Part print with two shaded views. Sizes in mm from the minimum x, y, z corner. Round coordinates to 2 decimals unless told otherwise and drop trailing zeros. Loops run counter-clockwise (first coordinate to the right, second up) from the corner with the lowest first, then second, coordinate; pieces in that order, holes last.
(1) Cut at A-A on y = 10. List the corners of the cut face in (x, z).
(2) Cut at D-D on y = 29. List the corners of the cut face in (x, z), then the cut area to 3 significant figures.
(3) Flat gauge pin, fed straight in: pin 1 (1 mm diameter, centred on y = 34, z = 2, fed in from +X). Where does the tip first touch, or does it go through?
(4) Mould opens along Y. For the marked faces 1, 2, 3 and 4 say: +Y half, -Y half, draft (parallel to the pull), parting line (faces both ways), or undercut.
(5) Cut at B-B on z = 2.85. Count the separate pieces of the cut face and the enclosed holes in it, then the cut area to 3 significant figures.
(6) Probe probe 1 along X at (y, z) = (12, 1.6); probe 2 along Y at (x, z) = (10, 2.85); probe 3 along Y at (x, z) = (16, 3.45). List the from-to ranges inside material, lowest first.
(7) Cut at C-C on x = 9.5. List the corners of the cut face in (y, z), then the cut area to 3 significant figures.
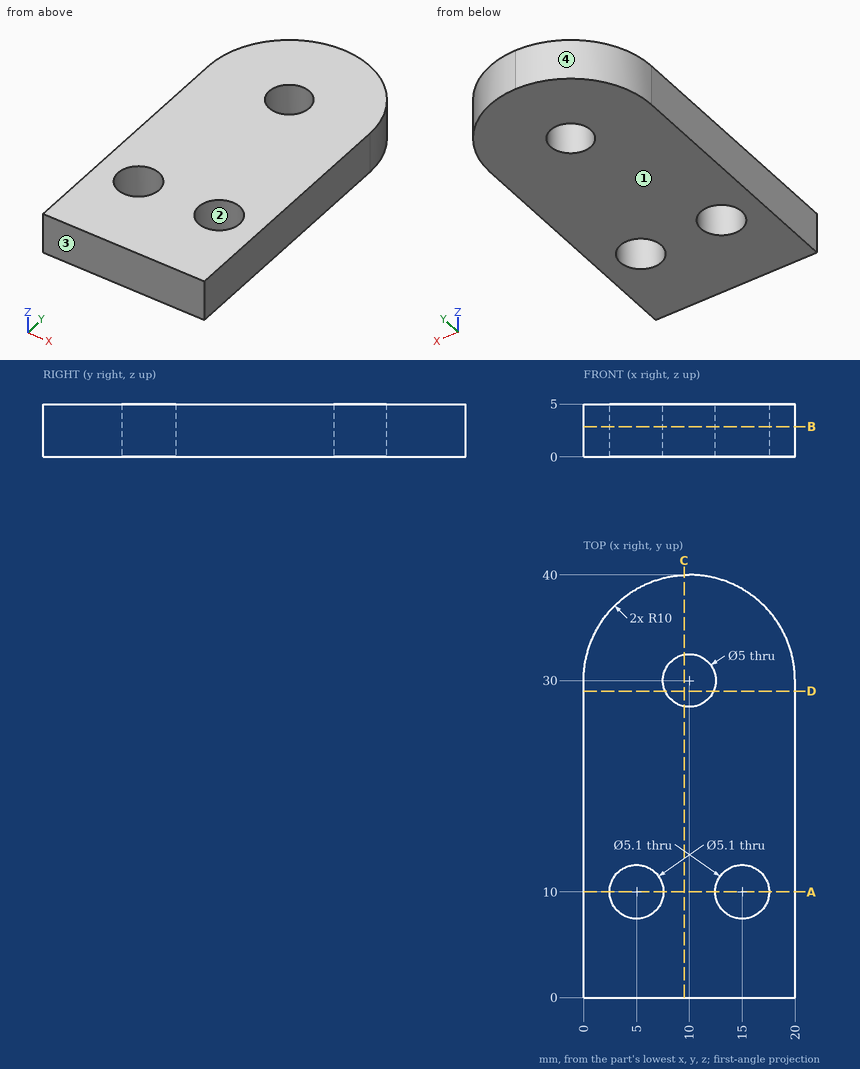
Final values:
1. outline: (0, 0) - (2.45, 0) - (2.45, 5) - (0, 5) - close; (7.55, 0) - (12.45, 0) - (12.45, 5) - (7.55, 5) - close; (17.55, 0) - (20, 0) - (20, 5) - (17.55, 5) - close
2. outline: (0, 0) - (7.71, 0) - (7.71, 5) - (0, 5) - close; (12.29, 0) - (20, 0) - (20, 5) - (12.29, 5) - close
2. area: 77.1 mm2
3. pin 1: stops at x = 19.37
4. face 1: draft
4. face 2: undercut
4. face 3: -Y half
4. face 4: +Y half
5. separate pieces: 1
5. enclosed holes: 3
5. area: 697 mm2
6. probe 1: x = 0 to 3.42, 6.58 to 13.42, 16.58 to 20
6. probe 2: y = 0 to 27.5, 32.5 to 40
6. probe 3: y = 0 to 7.65, 12.35 to 38
7. outline: (0, 0) - (27.55, 0) - (27.55, 5) - (0, 5) - close; (32.45, 0) - (39.99, 0) - (39.99, 5) - (32.45, 5) - close
7. area: 175 mm2
